The model under review builds one solid part; all positions refer to its coordinate system, in mm. Face numbers are marked on the shaded views. A direction names the side the tool comes from. Round coordinates to 2 decimals unless told otherwise and drop trailing zeros. Write each loop counter-clockwise with the first axis right and the second up, starting at its lowest first coordinate (ties: lowest second). Pieces come first, ordered by that corner, then holes. Notation, with made-up numbers: (41, 76) -> (62, 76) arc R20 ccw to (62, 104) -> close; hole circle Ø10 at (73.5, -27.5). An arc over 180 degrees is marked (long way). Answer as a JSON object with one key per item and string values. Group by question number.
1) Mouldability with a two-part tool opening along X and no side actions: class the marked faces 1, 2, 3 and 4 as pulls with the +X half, pulls with the -X half, needs draft (parallel to the pull), parting line crosses it, or undercut.
2) Insertion check: pin 1 Ø4 at (x, y) = (-14, 36.5) entering from -Z; pin 2 Ø1 at (x, z) = (-36.5, 1.5) entering from +Y; pin 3 Ø1.5 at (y, z) = (-5, -6.5) entering from -X. Each pin has a flat end and moves straight along its axis. Give the tip position at first contact, or say it passes through.
3) We need section C-C, the plane z = -0.5. Write out the cut boundary in (x, y).
4) To check wall thickness, follow probe 1 along X at (y, z) = (10, 5); probe 2 along Y at (x, z) = (-9, -6); probe 3 along Z at (x, y) = (-33.5, 29). State the ranges of each line that lie inside material, in increasing order. Write a range as [from, to].
5) Machinability: for the marked faces 5, 6 and 7, which of the approach directions +Z, -Z, +X, -X, +Y, -Y give a long, thin tool a straight path to every point of the face, cutting with its end or side? Answer none if there is none.
from build123d import *

# Parameters (mm, degrees)
BOSS_EXTRUDE1_DEPTH      = 10.5
BOSS_EXTRUDE1_DEPTH_BACK = 10.5
SKETCH1_R                = 8.25
SKETCH1_R_2              = 4.75
BOSS_EXTRUDE2_DEPTH      = 6.5
BOSS_EXTRUDE2_DEPTH_BACK = 6.5
SKETCH2_R                = 50
SKETCH2_R_2              = 40
BOSS_EXTRUDE3_DEPTH      = 2
BOSS_EXTRUDE3_DEPTH_BACK = 2
SKETCH3_R                = 40
SKETCH3_R_2              = 8.25
CHAMFER1_SIZE            = 4
FILLET1_R                = 3
REVOLVE1_ANGLE           = 45
CIRPATTERN1_COUNT        = 4
MIRROR1_COPY_1_ANGLE     = 45
MIRROR1_COPY_2_ANGLE     = 45
MIRROR1_COPY_3_ANGLE     = 45


# Read off the part's stored shape, not the designer's step: Revolve1
with BuildPart() as part:
    # Sketch1 → Boss-Extrude1 (new, two sides: drawn at the far end of the back side and taken through both)
    with BuildSketch(Plane.XY.offset(-BOSS_EXTRUDE1_DEPTH_BACK)):
        Circle(SKETCH1_R)
        Circle(SKETCH1_R_2, mode=Mode.SUBTRACT)
    extrude(amount=BOSS_EXTRUDE1_DEPTH + BOSS_EXTRUDE1_DEPTH_BACK)



with BuildPart() as body_2:
    # Sketch2 → Boss-Extrude2 (new, two sides: drawn at the far end of the back side and taken through both)
    with BuildSketch(Plane.XY.offset(-BOSS_EXTRUDE2_DEPTH_BACK)):
        Circle(SKETCH2_R)
        Circle(SKETCH2_R_2, mode=Mode.SUBTRACT)
    extrude(amount=BOSS_EXTRUDE2_DEPTH + BOSS_EXTRUDE2_DEPTH_BACK)


with BuildPart() as part_1:
    add(part.part)

    add(body_2.part)  # Boss-Extrude3 merges body 2
    # Sketch3 → Boss-Extrude3 (add, two sides: drawn at the far end of the back side and taken through both)
    with BuildSketch(Plane.XY.offset(-BOSS_EXTRUDE3_DEPTH_BACK)):
        Circle(SKETCH3_R)
        Circle(SKETCH3_R_2, mode=Mode.SUBTRACT)
    extrude(amount=BOSS_EXTRUDE3_DEPTH + BOSS_EXTRUDE3_DEPTH_BACK)

    # Chamfer1
    chamfer1_edges = [part_1.edges().sort_by_distance(p)[0] for p in [
        (-40, 0, -2),
        (-40, 0, 2),
    ]]
    chamfer(chamfer1_edges, length=CHAMFER1_SIZE)

    # Fillet1
    fillet1_edges = [part_1.edges().sort_by_distance(p)[0] for p in [
        (-50, 0, -6.5),
        (-50, 0, 6.5),
    ]]
    fillet(fillet1_edges, radius=FILLET1_R)

    # Revolve1 outline → Revolve1 (revolve)
    with BuildSketch(Plane(origin=(0, 0, 0), x_dir=(-0.9238795325112862, 0.3826834323650911, 0), z_dir=(0.3826834323650911, 0.9238795325112862, 0))):
        Polygon((36, 2), (8.25, 8.5), (8.25, 2), align=None)
    revolve1 = revolve(axis=Axis((0, 0, 0), (0, 0, 1)), revolution_arc=REVOLVE1_ANGLE)

    # CirPattern1: Revolve1 ×4 about axis
    cirpattern1_axis = Axis((0, 0, -10.5), (0, 0, 1))
    for i in range(1, CIRPATTERN1_COUNT):
        add(revolve1.rotate(cirpattern1_axis, i * 360 / CIRPATTERN1_COUNT))

    # Mirror1: Revolve1 across plane
    add(revolve1.mirror(Plane.XY))

    # Mirror1 copy 1 sketch → Mirror1 copy 1 (revolve)
    with BuildSketch(Plane(origin=(0, 0, 0), x_dir=(-0.38268343236509117, -0.9238795325112862, 0), z_dir=(-0.9238795325112862, 0.38268343236509117, 0))):
        Polygon((36, -2), (8.25, -8.5), (8.25, -2), align=None)
    revolve(axis=Axis((0, 0, 0), (0, 0, 1)), revolution_arc=MIRROR1_COPY_1_ANGLE)

    # Mirror1 copy 2 sketch → Mirror1 copy 2 (revolve)
    with BuildSketch(Plane(origin=(0, 0, 0), x_dir=(0.9238795325112862, -0.3826834323650912, 0), z_dir=(-0.3826834323650912, -0.9238795325112862, 0))):
        Polygon((36, -2), (8.25, -8.5), (8.25, -2), align=None)
    revolve(axis=Axis((0, 0, 0), (0, 0, 1)), revolution_arc=MIRROR1_COPY_2_ANGLE)

    # Mirror1 copy 3 sketch → Mirror1 copy 3 (revolve)
    with BuildSketch(Plane(origin=(0, 0, 0), x_dir=(0.3826834323650913, 0.9238795325112861, 0), z_dir=(0.9238795325112861, -0.3826834323650913, 0))):
        Polygon((36, -2), (8.25, -8.5), (8.25, -2), align=None)
    revolve(axis=Axis((0, 0, 0), (0, 0, 1)), revolution_arc=MIRROR1_COPY_3_ANGLE)


solid = part_1.part
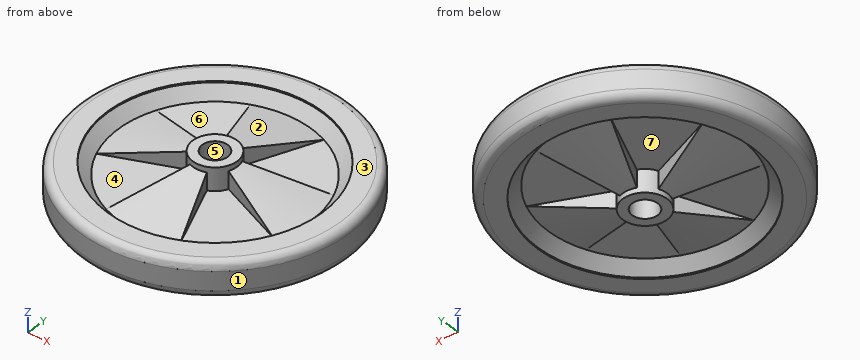
Here are the results:
{
 "1": {"face 1": "parting line crosses it", "face 2": "undercut", "face 3": "needs draft", "face 4": "undercut"},
 "2": {"pin 1": "stops at z = -6.5", "pin 2": "stops at y = 34.7", "pin 3": "stops at x = -48.73"},
 "3": {"outline": "circle Ø100 at (0, 0); hole circle Ø9.5 at (0, 0)"},
 "4": {"probe 1": "x = [-48.58, -37.7], [-4.14, 4.14], [37.7, 48.58]", "probe 2": "y = [-47.82, -38.97], [-3.73, 3.73], [38.97, 47.82]", "probe 3": "z = [-6.5, 6.5]"},
 "5": {"face 5": "+Z, -Z", "face 6": "+Z", "face 7": "-Z"}
}
